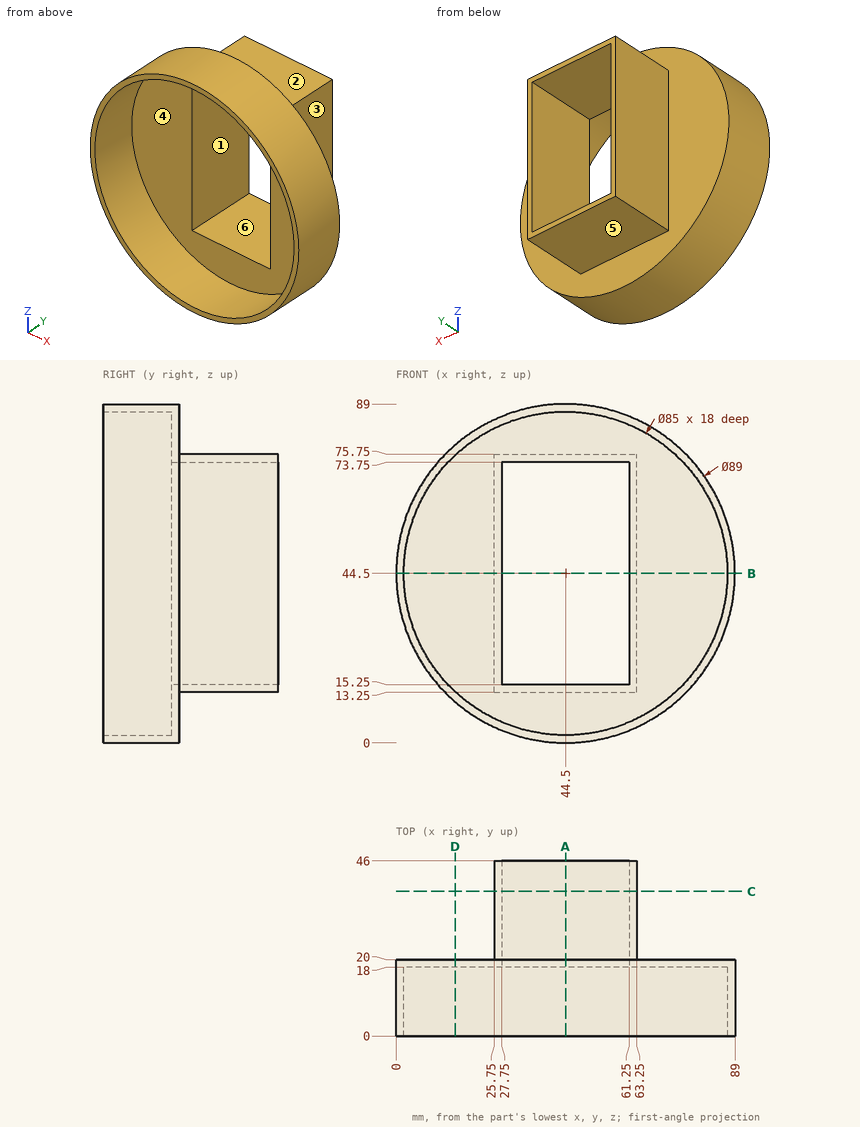
For this review, use the dimensioned drawing (mm, ordinates from the lowest corner) and the shaded views. A direction names the side the tool comes from. Give positions to 0.01 mm unless a question says otherwise; leave off trailing zeros. Order: outer loops, then holes, each group sorted by start corner. A loop starts at its lowest first (then second) coordinate and runs counter-clockwise, first axis right, second up. Notation, with made-up numbers: (55.25, -10.75) - (69.25, -10.75) arc R15 ccw to (69.25, -1.75) - close; hole circle Ø5 at (62, 25). An arc over 180 degrees is marked (long way). Use CSV: the item, a comma, the result in double quotes. Start each with the question number.
Q1. Draft analysis for pull direction X (two halves, no side actions). For the marked faces 1, 2 and 3, state which applies: pulls with the +X half, pulls with the -X half, needs draft (parallel to the pull), parting line crosses it, or undercut.
Q2. Take a section at C-C (y = 38). State the section outline as (x, z) points, and give its area (3 significant figures).
Q3. For P1, Ø5, axis at x = 51, y = 41, coming from the -Z side; P2, Ø4, axis at y = 19, z = 79.5, coming from the +X side; P3, Ø5, axis at x = 57.5, z = 52, coming from the -Y side; P4, Ø5, axis at x = 70, z = 56, coming from the -Y side, all flat-tipped, find the tip position at first contact; note any pin that passes through.
Q4. Machinability: for the marked faces 4, 5 and 6, which of the approach directions +Z, -Z, +X, -X, +Y, -Y give a long, thin tool a straight path to every point of the face, cutting with its end or side? Answer none if there is none.
Q5. Take a section at B-B (z = 44.5). State the section outline as (x, y) points, and give its area (3 significant figures).
Q6. Take a section at A-A (x = 44.5). State the section outline as (y, z) points.
Q7. Take a section at D-D (x = 15.5). State the section outline as (y, z) points.
Q8. For line 1 (Z direction, x = 44, y = 5); line 2 (Z direction, x = 58.5, y = 28); line 3 (X direction, y = 37, z = 17), list the stretches that pass through material, from the lowest coordinate up.
Calculated:
1,face 1,"undercut"
1,face 2,"needs draft"
1,face 3,"pulls with the +X half"
2,outline,"(25.75, 13.25) - (63.25, 13.25) - (63.25, 75.75) - (25.75, 75.75) - close; hole (27.75, 15.25) - (61.25, 15.25) - (61.25, 73.75) - (27.75, 73.75) - close"
2,area,"384 mm²"
3,P1,"stops at z = 13.25"
3,P2,"stops at x = 74.35"
3,P3,"passes through"
3,P4,"stops at y = 18"
4,face 4,"-Y"
4,face 5,"-Z, +X, -X, +Y"
4,face 6,"+Y, -Y"
5,outline,"(0, 0) - (2, 0) - (2, 18) - (27.75, 18) - (27.75, 46) - (25.75, 46) - (25.75, 20) - (0, 20) - close; (61.25, 18) - (87, 18) - (87, 0) - (89, 0) - (89, 20) - (63.25, 20) - (63.25, 46) - (61.25, 46) - close"
5,area,"287 mm²"
6,outline,"(0, 0) - (20, 0) - (20, 13.25) - (46, 13.25) - (46, 15.25) - (18, 15.25) - (18, 2) - (0, 2) - close; (0, 87) - (18, 87) - (18, 73.75) - (46, 73.75) - (46, 75.75) - (20, 75.75) - (20, 89) - (0, 89) - close"
7,outline,"(0, 10.75) - (20, 10.75) - (20, 78.25) - (0, 78.25) - (0, 75.57) - (18, 75.57) - (18, 13.43) - (0, 13.43) - close"
8,line 1,"z = 0 to 2, 87 to 89"
8,line 2,"z = 13.25 to 15.25, 73.75 to 75.75"
8,line 3,"x = 25.75 to 27.75, 61.25 to 63.25"
